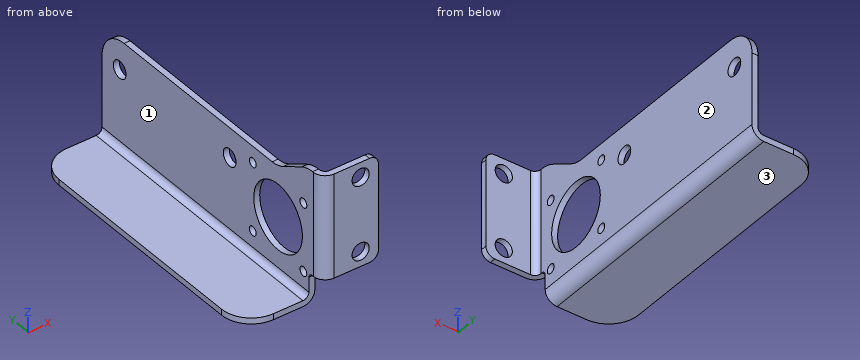
```python
from build123d import *

# Parameters (mm, degrees)
BASE_FLANGE1_DEPTH     = 17.5
M5_CLEARANCE_HOLE2_D   = 5.8
M5_CLEARANCE_HOLE1_D   = 5.8
BOSS_EXTRUDE1_DEPTH    = 2
M2_5_CLEARANCE_HOLE1_D = 3.1
SKETCH13_R             = 11.05
CUT_EXTRUDE2_DEPTH     = 10
SKETCH16_W             = 3.5
SKETCH16_H             = 66
BOSS_EXTRUDE2_DEPTH    = 2
EDGE_FLANGE1_DEPTH     = 94
CUT_EXTRUDE3_DEPTH     = 2
FILLET1_R              = 10
FILLET2_R              = 3
FILLET3_R              = 1.5


# Sheet-metal steps are written as plain solids
with BuildPart() as part:
    # Sketch1 → Base-Flange1 (new, symmetric)
    with BuildSketch(Plane.XY):
        with BuildLine():
            Line((0, 100), (0, 4))
            ThreePointArc((0, 4), (1.171572875, 1.171572875), (4, 0))
            Line((4, 0), (19, 0))
            Line((19, 0), (19, 2))
            Line((19, 2), (4, 2))
            ThreePointArc((4, 2), (2.585786438, 2.585786438), (2, 4))
            Line((2, 4), (2, 100))
            Line((2, 100), (0, 100))
        make_face()
    extrude(amount=BASE_FLANGE1_DEPTH, both=True)

    # M5 Clearance Hole2 (through all)
    with Locations(Plane(origin=(0, 2, 0), x_dir=(1, 0, 0), z_dir=(0, 1, 0))):
        with Locations((13, -12.5), (13, 12.5)):
            Hole(M5_CLEARANCE_HOLE2_D / 2)

    # M5 Clearance Hole1 (through all)
    with Locations(Plane(origin=(2, 0, 0), x_dir=(0, 0, -1), z_dir=(1, 0, 0))):
        with Locations((0, 92), (0, 42)):
            Hole(M5_CLEARANCE_HOLE1_D / 2)

    # Sketch12 → Boss-Extrude1 (add)
    with BuildSketch(Plane(origin=(2, 0, 0), x_dir=(0, 0, -1), z_dir=(1, 0, 0))):
        Polygon((16.892359744, 6), (21, 6), (21, 34), (14.5, 34), align=None)
    extrude(amount=-BOSS_EXTRUDE1_DEPTH)

    # M2.5 Clearance Hole1 (through all)
    with Locations(Plane(origin=(2, 0, 0), x_dir=(0, 0, -1), z_dir=(1, 0, 0))):
        with Locations((18.5, 8.5), (-4.5, 8.5), (-4.5, 31.5), (18.5, 31.5)):
            Hole(M2_5_CLEARANCE_HOLE1_D / 2)

    # Sketch13 → Cut-Extrude2 (cut)
    with BuildSketch(Plane(origin=(2, 0, 0), x_dir=(0, 0, -1), z_dir=(1, 0, 0))):
        with Locations(Location((7, 20, 0), (0, 0, 90))):
            Circle(SKETCH13_R)
    extrude(amount=-CUT_EXTRUDE2_DEPTH, mode=Mode.SUBTRACT)

    # Sketch16 → Boss-Extrude2 (add)
    with BuildSketch(Plane(origin=(2, 0, 0), x_dir=(0, 0, -1), z_dir=(1, 0, 0))):
        with Locations((19.25, 67)):
            Rectangle(SKETCH16_W, SKETCH16_H)
    extrude(amount=-BOSS_EXTRUDE2_DEPTH)

    # Edge-Flange1 section (across the edge) → Edge-Flange1 (add)
    with BuildSketch(Plane(origin=(0, 100, -26), x_dir=(0, 0, 1), z_dir=(0, -1, 0))):
        with BuildLine():
            Line((-2, 2), (-2, 22))
            Line((-2, 22), (0, 22))
            Line((0, 22), (0, 2))
            ThreePointArc((0, 2), (0.585786438, 0.585786438), (2, 0))
            Line((2, 0), (5, 0))
            Line((5, 0), (5, -2))
            Line((5, -2), (2, -2))
            ThreePointArc((2, -2), (-0.828427125, -0.828427125), (-2, 2))
        make_face()
    extrude(amount=EDGE_FLANGE1_DEPTH)

    # Sketch20 → Cut-Extrude3 (cut)
    with BuildSketch(Plane(origin=(2, 0, 0), x_dir=(0, 0, -1), z_dir=(1, 0, 0))):
        Polygon((-10, 100), (-10, 19.990381057), (-17.5, 7), (-17.5, 100), align=None)
    extrude(amount=-CUT_EXTRUDE3_DEPTH, mode=Mode.SUBTRACT)

    # Fillet1
    fillet1_edges = [part.edges().sort_by_distance(p)[0] for p in [
        (-22, 100, -27),
        (-22, 6, -27),
        (1, 100, 10),
        (1, 19.990381057, 10),
        (1, 7, 17.5),
    ]]
    fillet(fillet1_edges, radius=FILLET1_R)

    # Fillet2
    fillet2_edges = [part.edges().sort_by_distance(p)[0] for p in [
        (19, 1, 17.5),
        (19, 1, -17.5),
    ]]
    fillet(fillet2_edges, radius=FILLET2_R)

    # Fillet3
    fillet3_edges = [part.edges().sort_by_distance(p)[0] for p in [
        (1, 6, -17.5),
    ]]
    fillet(fillet3_edges, radius=FILLET3_R)


solid = part.part
```
Verification items for the finished model (mm, model axes). Face numbers are marked on the shaded views. A direction names the side the tool comes from. Round coordinates to 2 decimals unless told otherwise and drop trailing zeros. Write each loop counter-clockwise with the first axis right and the second up, starting at its lowest first coordinate (ties: lowest second). Pieces come first, ordered by that corner, then holes.
1. Section check B-B on z = -7. Enter the section's corners in (x, y).
2. Section check C-C on x = 12. Enter the section's corners in (y, z).
3. Section check D-D on z = -12.5. Enter the section's corners in (x, y).
4. Scan lines: L1, parallel to Z at x = 13, y = 0.6; L2, parallel to X at y = 74.5, z = -14. Record each from-to range of solid material in increasing order.
5. Section check A-A on y = 42. Enter the section's corners in (x, z), plus the area to 3 significant figures.
6. Access from +Z, -Z, +X, -X, +Y, -Y to the whole of each face (thin tool, end or side, straight path). Record for the marked faces 1, 2 and 3.
7. Gauge pin test, flat ends, axial feed: P1, Ø2, axis at x = 1, y = 45.5, coming from the +Z side; P2, Ø16, axis at x = -15, y = 40, coming from the +Z side; P3, Ø12, axis at x = 0.5, y = 31.5, coming from the -Z side; P4, Ø16.5, axis at x = 15, z = -3, coming from the +Y side. Record the tip position at first contact, or that the pin passes through.
Answer:
1. outline: (0, 4) arc R4 ccw to (4, 0) - (19, 0) - (19, 2) - (4, 2) arc R2 cw to (2, 4) - (2, 8.95) - (0, 8.95) - close; (0, 31.05) - (2, 31.05) - (2, 100) - (0, 100) - close
2. outline: (0, -17.5) - (2, -17.5) - (2, -15.22) - (0, -15.22) - close; (0, -9.78) - (2, -9.78) - (2, 9.78) - (0, 9.78) - close; (0, 15.22) - (2, 15.22) - (2, 17.5) - (0, 17.5) - close
3. outline: (0, 4) arc R4 ccw to (4, 0) - (10.1, 0) - (10.1, 2) - (4, 2) arc R2 cw to (2, 4) - (2, 10.42) - (0, 10.42) - close; (0, 29.58) - (2, 29.58) - (2, 100) - (0, 100) - close; (15.9, 0) - (19, 0) - (19, 2) - (15.9, 2) - close
4. L1: z = -17.5 to -15.4, -9.6 to 9.6, 15.4 to 17.5
4. L2: x = 0 to 2
5. outline: (-22, -28) - (-2, -28) arc R4 ccw to (2, -24) - (2, -2.9) - (0, -2.9) - (0, -24) arc R2 cw to (-2, -26) - (-22, -26) - close; (0, 2.9) - (2, 2.9) - (2, 10) - (0, 10) - close
5. area: 106 mm2
6. face 1: +Z, -X, +Y, -Y
6. face 2: +Z, -Z, +X, +Y
6. face 3: -Z, +X, -X, +Y, -Y
7. P1: stops at z = 10
7. P2: stops at z = -26
7. P3: stops at z = -28
7. P4: stops at y = 2
